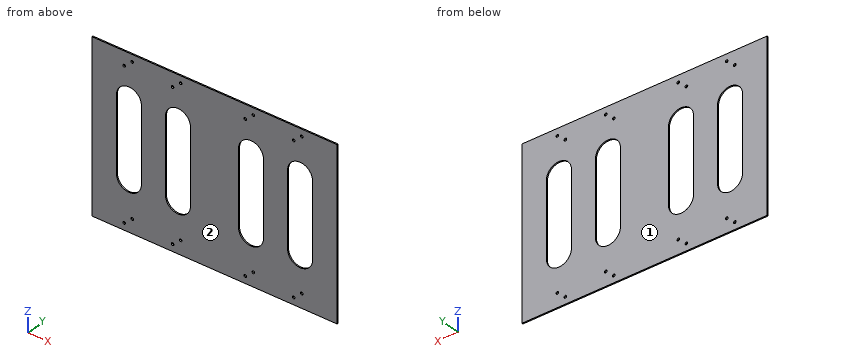
from build123d import *

# Parameters (mm, degrees)
SKETCH1_W                 = 392
SKETCH1_H                 = 272
BOSS_EXTRUDE1_DEPTH       = 2
CUT_EXTRUDE1_REACH        = 240.571
SKETCH2_R                 = 2.125
LPATTERN1_COUNT           = 2
LPATTERN1_PITCH           = 77.4
LPATTERN7_COUNT           = 2
LPATTERN7_PITCH           = 193.5
LPATTERN7_COPY_1_REACH    = 240.571
LPATTERN7_COPY_1_SKETCH_R = 2.125
CUT_EXTRUDE2_DEPTH        = 239.570744225


with BuildPart() as part:
    # Sketch1 → Boss-Extrude1 (new body)
    with BuildSketch(Plane(origin=(0, 0, 0), x_dir=(1, 0, 0), z_dir=(0, 1, 0))):
        Rectangle(SKETCH1_W, SKETCH1_H)
    extrude(amount=BOSS_EXTRUDE1_DEPTH)

    # Sketch2 → Cut-Extrude1 (cut, up to next)
    with BuildSketch(Plane(origin=(0, 2, 0), x_dir=(1, 0, 0), z_dir=(0, 1, 0)), mode=Mode.PRIVATE) as cut_extrude1_sk1:
        with Locations(Location((139.4, -124.77, 0), (0, 0, 270))):
            Circle(SKETCH2_R)
    cut_extrude1_tool1 = extrude(cut_extrude1_sk1.sketch, amount=-CUT_EXTRUDE1_REACH, mode=Mode.PRIVATE) & part.part
    # Sketch2 → Cut-Extrude1 (cut, up to next)
    with BuildSketch(Plane(origin=(0, 2, 0), x_dir=(1, 0, 0), z_dir=(0, 1, 0)), mode=Mode.PRIVATE) as cut_extrude1_sk2:
        with Locations(Location((126.5, -113.53, 0), (0, 0, 270))):
            Circle(SKETCH2_R)
    cut_extrude1_tool2 = extrude(cut_extrude1_sk2.sketch, amount=-CUT_EXTRUDE1_REACH, mode=Mode.PRIVATE) & part.part
    # Sketch2 → Cut-Extrude1 (cut, up to next)
    with BuildSketch(Plane(origin=(0, 2, 0), x_dir=(1, 0, 0), z_dir=(0, 1, 0)), mode=Mode.PRIVATE) as cut_extrude1_sk3:
        with Locations(Location((126.5, 124.77, 0), (0, 0, 270))):
            Circle(SKETCH2_R)
    cut_extrude1_tool3 = extrude(cut_extrude1_sk3.sketch, amount=-CUT_EXTRUDE1_REACH, mode=Mode.PRIVATE) & part.part
    # Sketch2 → Cut-Extrude1 (cut, up to next)
    with BuildSketch(Plane(origin=(0, 2, 0), x_dir=(1, 0, 0), z_dir=(0, 1, 0)), mode=Mode.PRIVATE) as cut_extrude1_sk4:
        with Locations(Location((139.4, 113.53, 0), (0, 0, 270))):
            Circle(SKETCH2_R)
    cut_extrude1_tool4 = extrude(cut_extrude1_sk4.sketch, amount=-CUT_EXTRUDE1_REACH, mode=Mode.PRIVATE) & part.part
    cut_extrude1_1 = cut_extrude1_tool1.solids().sort_by_distance((139.4, 2, 124.77))[0]
    add(cut_extrude1_1, mode=Mode.SUBTRACT)
    cut_extrude1_2 = cut_extrude1_tool2.solids().sort_by_distance((126.5, 2, 113.53))[0]
    add(cut_extrude1_2, mode=Mode.SUBTRACT)
    cut_extrude1_3 = cut_extrude1_tool3.solids().sort_by_distance((126.5, 2, -124.77))[0]
    add(cut_extrude1_3, mode=Mode.SUBTRACT)
    cut_extrude1_4 = cut_extrude1_tool4.solids().sort_by_distance((139.4, 2, -113.53))[0]
    add(cut_extrude1_4, mode=Mode.SUBTRACT)
    cut_extrude1 = cut_extrude1_1 + cut_extrude1_2 + cut_extrude1_3 + cut_extrude1_4  # Cut-Extrude1 as one shape, for the pattern or mirror that repeats it

    # LPattern1: Cut-Extrude1 ×2
    with Locations(*[(-i * LPATTERN1_PITCH, 0, 0) for i in range(1, LPATTERN1_COUNT)]):
        add(cut_extrude1, mode=Mode.SUBTRACT)

    # LPattern7: Cut-Extrude1 ×2
    with Locations(*[(-i * LPATTERN7_PITCH, 0, 0) for i in range(1, LPATTERN7_COUNT)]):
        add(cut_extrude1, mode=Mode.SUBTRACT)

    # LPattern7 copy 1 sketch → LPattern7 copy 1 (cut, up to next)
    with BuildSketch(Plane(origin=(-270.9, 2, 0), x_dir=(1, 0, 0), z_dir=(0, 1, 0)), mode=Mode.PRIVATE) as lpattern7_copy_1_sk1:
        with Locations(Location((139.4, -124.77, 0), (0, 0, 270))):
            Circle(LPATTERN7_COPY_1_SKETCH_R)
    lpattern7_copy_1_tool1 = extrude(lpattern7_copy_1_sk1.sketch, amount=-LPATTERN7_COPY_1_REACH, mode=Mode.PRIVATE) & part.part
    # LPattern7 copy 1 sketch → LPattern7 copy 1 (cut, up to next)
    with BuildSketch(Plane(origin=(-270.9, 2, 0), x_dir=(1, 0, 0), z_dir=(0, 1, 0)), mode=Mode.PRIVATE) as lpattern7_copy_1_sk2:
        with Locations(Location((126.5, -113.53, 0), (0, 0, 270))):
            Circle(LPATTERN7_COPY_1_SKETCH_R)
    lpattern7_copy_1_tool2 = extrude(lpattern7_copy_1_sk2.sketch, amount=-LPATTERN7_COPY_1_REACH, mode=Mode.PRIVATE) & part.part
    # LPattern7 copy 1 sketch → LPattern7 copy 1 (cut, up to next)
    with BuildSketch(Plane(origin=(-270.9, 2, 0), x_dir=(1, 0, 0), z_dir=(0, 1, 0)), mode=Mode.PRIVATE) as lpattern7_copy_1_sk3:
        with Locations(Location((126.5, 124.77, 0), (0, 0, 270))):
            Circle(LPATTERN7_COPY_1_SKETCH_R)
    lpattern7_copy_1_tool3 = extrude(lpattern7_copy_1_sk3.sketch, amount=-LPATTERN7_COPY_1_REACH, mode=Mode.PRIVATE) & part.part
    # LPattern7 copy 1 sketch → LPattern7 copy 1 (cut, up to next)
    with BuildSketch(Plane(origin=(-270.9, 2, 0), x_dir=(1, 0, 0), z_dir=(0, 1, 0)), mode=Mode.PRIVATE) as lpattern7_copy_1_sk4:
        with Locations(Location((139.4, 113.53, 0), (0, 0, 270))):
            Circle(LPATTERN7_COPY_1_SKETCH_R)
    lpattern7_copy_1_tool4 = extrude(lpattern7_copy_1_sk4.sketch, amount=-LPATTERN7_COPY_1_REACH, mode=Mode.PRIVATE) & part.part
    add(lpattern7_copy_1_tool1.solids().sort_by_distance((-131.5, 2, 124.77))[0], mode=Mode.SUBTRACT)
    add(lpattern7_copy_1_tool2.solids().sort_by_distance((-144.4, 2, 113.53))[0], mode=Mode.SUBTRACT)
    add(lpattern7_copy_1_tool3.solids().sort_by_distance((-144.4, 2, -124.77))[0], mode=Mode.SUBTRACT)
    add(lpattern7_copy_1_tool4.solids().sort_by_distance((-131.5, 2, -113.53))[0], mode=Mode.SUBTRACT)

    # Sketch3 → Cut-Extrude2 (cut, through all)
    with BuildSketch(Plane(origin=(0, 2, 0), x_dir=(1, 0, 0), z_dir=(0, 1, 0))):
        with BuildLine():
            Line((-116.8, 55.364791438), (-116.8, -64.635208562))
            ThreePointArc((-116.8, -64.635208562), (-136.8, -84.635208562), (-156.8, -64.635208562))
            Line((-156.8, -64.635208562), (-156.8, 55.364791438))
            ThreePointArc((-156.8, 55.364791438), (-136.8, 75.364791438), (-116.8, 55.364791438))
        make_face()
        with BuildLine():
            Line((-38.4, 55.364791438), (-38.4, -64.635208562))
            ThreePointArc((-38.4, -64.635208562), (-58.4, -84.635208562), (-78.4, -64.635208562))
            Line((-78.4, -64.635208562), (-78.4, 55.364791438))
            ThreePointArc((-78.4, 55.364791438), (-58.4, 75.364791438), (-38.4, 55.364791438))
        make_face()
        with BuildLine():
            Line((38.4, 55.364791438), (38.4, -64.635208562))
            ThreePointArc((38.4, -64.635208562), (58.4, -84.635208562), (78.4, -64.635208562))
            Line((78.4, -64.635208562), (78.4, 55.364791438))
            ThreePointArc((78.4, 55.364791438), (58.4, 75.364791438), (38.4, 55.364791438))
        make_face()
        with BuildLine():
            Line((116.8, 55.364791438), (116.8, -64.635208562))
            ThreePointArc((116.8, -64.635208562), (136.8, -84.635208562), (156.8, -64.635208562))
            Line((156.8, -64.635208562), (156.8, 55.364791438))
            ThreePointArc((156.8, 55.364791438), (136.8, 75.364791438), (116.8, 55.364791438))
        make_face()
    extrude(amount=-CUT_EXTRUDE2_DEPTH, mode=Mode.SUBTRACT)


solid = part.part
Build history of the part. All positions in model axes, mm. Face numbers are marked on the shaded views. Round coordinates to 2 decimals unless told otherwise and drop trailing zeros. Write each loop counter-clockwise with the first axis right and the second up, starting at its lowest first coordinate (ties: lowest second). Pieces come first, ordered by that corner, then holes. Notation, with made-up numbers: (77, 80.5) -> (133, 80.5) arc R24 cw to (133, 91.5) -> close; hole circle Ø11 at (31.25, 39). An arc over 180 degrees is marked (long way). Write item = value, one per line.
(1) Flat gauge pin, fed straight in: pin 1 (3.5 mm diameter, centred on x = 139.4, z = -113.53, fed in from -Y). Where does the tip first touch, or does it go through?
Answer:
pin_1 = through
(2) Band-saw the part on B-B (x = -124.5). Give the cut face in (y, z).
Answer:
outline = (0, -136) -> (2, -136) -> (2, -71.14) -> (0, -71.14) -> close; (0, 80.41) -> (2, 80.41) -> (2, 136) -> (0, 136) -> close
(3) Band-saw the part on A-A (z = -47.5). Give the cut face in (x, y), then the cut area to 3 significant figures.
Answer:
outline = (-196, 0) -> (-156.8, 0) -> (-156.8, 2) -> (-196, 2) -> close; (-116.8, 0) -> (-78.4, 0) -> (-78.4, 2) -> (-116.8, 2) -> close; (-38.4, 0) -> (38.4, 0) -> (38.4, 2) -> (-38.4, 2) -> close; (78.4, 0) -> (116.8, 0) -> (116.8, 2) -> (78.4, 2) -> close; (156.8, 0) -> (196, 0) -> (196, 2) -> (156.8, 2) -> close
area = 464 mm2
(4) Band-saw the part on C-C (y = 0.9). State how many separate pieces and enclosed holes the cut face has, then the cut area to 3 significant figures.
Answer:
separate_pieces = 1
enclosed_holes = 20
area = 82,200 mm2
(5) Probe L1, parallel to X at y = 1.6, z = 49; L2, parallel to X at y = 1.35, z = -124.77 (3 decimals); L3, parallel to Z at x = 127, y = 0.45. List the from-to ranges inside material, lowest first.
Answer:
L1 = -196 to -156.8, -116.8 to -78.4, -38.4 to 38.4, 78.4 to 116.8, 156.8 to 196
L2 = -196 to -146.525, -142.275 to -69.125, -64.875 to 46.975, 51.225 to 124.375, 128.625 to 196
L3 = -136 to -126.84, -122.7 to -72.8, 82.07 to 111.46, 115.6 to 136
(6) Band-saw the part on D-D (z = 79.5). Give the cut face in (x, y).
Answer:
outline = (-196, 0) -> (-150.18, 0) -> (-150.18, 2) -> (-196, 2) -> close; (-123.42, 0) -> (-71.78, 0) -> (-71.78, 2) -> (-123.42, 2) -> close; (-45.02, 0) -> (45.02, 0) -> (45.02, 2) -> (-45.02, 2) -> close; (71.78, 0) -> (123.42, 0) -> (123.42, 2) -> (71.78, 2) -> close; (150.18, 0) -> (196, 0) -> (196, 2) -> (150.18, 2) -> close
(7) Two-plate mould, pull along Y, no slides. Class the marked faces 1 and 2: pulls with the +Y half, pulls with the -Y half, needs draft (parallel to the pull), parting line crosses it, or undercut.
Answer:
face_1 = pulls with the +Y half
face_2 = pulls with the -Y half
